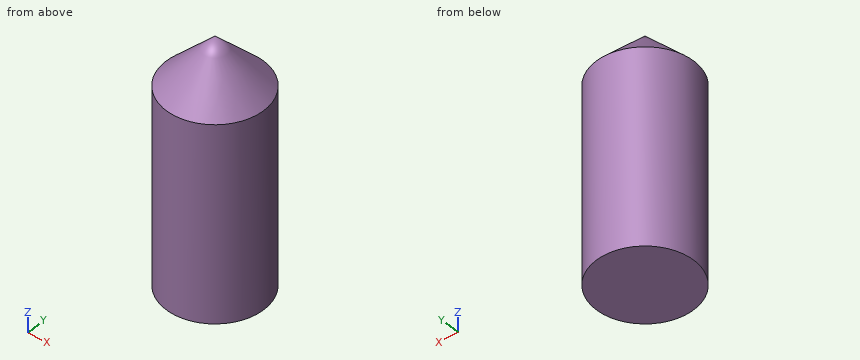
from build123d import *

# Parameters (mm, degrees)
F0_R     = 12.7
F1_DEPTH = 50.8
F2_R     = 10.16
F3_DEPTH = 48.26
F4_R     = 12.7
F5_DEPTH = 25.4
F5_TAPER = 45


with BuildPart() as f1:
    # F0 (on Top) → F1 (new body)
    with BuildSketch(Plane.XY):
        Circle(F0_R)
    extrude(amount=F1_DEPTH)

    # F2 (on face) → F3 (cut)
    with BuildSketch(Plane.XY.offset(50.8)):
        Circle(F2_R)
    extrude(amount=-F3_DEPTH, mode=Mode.SUBTRACT)

    # F4 (on face) → F5 (join)
    with BuildSketch(Plane.XY.offset(50.8)):
        Circle(F4_R)
    extrude(amount=F5_DEPTH, taper=F5_TAPER)


solid = f1.part
Source: CAD feature listing. Evaluate the final solid. Frame: model axes, mm. Give positions to 0.01 mm unless a question says otherwise; leave off trailing zeros. Order: outer loops, then holes, each group sorted by start corner. A loop starts at its lowest first (then second) coordinate and runs counter-clockwise, first axis right, second up. Notation, with made-up numbers: (63.5, 55.25) -> (90.5, 55.25) arc R24 cw to (90.5, 83.25) -> close; hole circle Ø4 at (10.25, 39.5). An arc over 180 degrees is marked (long way). Use a Markdown table: item, result.
1) Ray query, line 1 along Y through (x, z) = (-0.25, 38.5); line 2 along Y through (x, z) = (0.5, 27.5). Return the intervals inside material, ascending. Write a range as [from, to].
Answer list:
| item | result |
|---|---|
| line 1 | [-12.7, -10.16], [10.16, 12.7] |
| line 2 | [-12.69, -10.15], [10.15, 12.69] |
2) Contact query for flat-ended pins moving along their axis: P1, Ø3, axis at y = 5.5, z = 46.5, coming from the +X side; P2, Ø1.5, axis at x = -5, y = 4.5, coming from the +Z side; P3, Ø5, axis at x = 0, z = 53.5, coming from the -Y side. Output: stop coordinate, or through.
Answer list:
| item | result |
|---|---|
| P1 | x = 12.05 |
| P2 | z = 57.52 |
| P3 | y = -12.5 |
3) Section query A-A, the plane z = 34. Return the cut outline in (x, y).
Answer list:
| item | result |
|---|---|
| outline | circle Ø25.4 at (0, 0); hole circle Ø20.32 at (0, 0) |
